Autodesk Inventor part; units mm, degrees
ref_plane "YZ Plane" through (0, 0, 0) normal (1, 0, 0) x (0, 1, 0)
ref_plane "XZ Plane" through (0, 0, 0) normal (0, 1, 0) x (-1, 0, 0)
ref_plane "XY Plane" through (0, 0, 0) normal (0, 0, 1) x (1, 0, 0)
sketch "Sketch1" plane through (0, 0, 0) normal (0, 0, 1) x (1, 0, 0)
  line L0 (50, -70) -> (50, 25)
  line L1 (-50, 25) -> (-50, -70)
  line L2 (0, 0) -> (-38.1854, 57.2781) construction
  arc A0 (50, 25) -> (-50, 25) centre (0, 25) ccw
  line L3 (-45, -90) -> (45, -90)
  line L4 (0, 0) -> (38.1854, 57.2781) construction
  line L5 (50, -70) -> (50, -85)
  line L6 (-50, -70) -> (-50, -85)
  arc A1 (45, -90) -> (50, -85) centre (45, -85) ccw
  arc A2 (-50, -85) -> (-45, -90) centre (-45, -85) ccw
  dimension "d19" = 5
extrude "Extrusion1" add sketch "Sketch1" along normal blind 47.5
shell "Shell1" thickness 2.5 removed faces 1 at (-16.6667, -6.6667, 0)
sketch "Sketch2" plane through (0, 25, 45) normal (0, 0, -1) x (-1, 0, 0)
  arc A0 (50, 0) -> (-50, 0) centre (0, 0) ccw
  line L0 (25, 0) -> (50, 0) construction
  line L1 (25, 0) -> (50, 0) construction
  line L2 (-25, 0) -> (-50, 0)
  line L3 (-47.5, -110) -> (-47.5, 0)
  line L4 (25, 0) -> (50, 0) construction
  line L5 (25, 0) -> (50, 0) construction
  line L6 (47.5, 0) -> (47.5, -112.5)
  line L7 (47.5, -112.5) -> (-47.5, -112.5)
  line L8 (-47.5, -112.5) -> (-47.5, 0)
  line L9 (20.5, -24.5) -> (29.5, -24.5)
  line L10 (29.5, -24.5) -> (29.5, -15.5)
  line L11 (29.5, -15.5) -> (20.5, -15.5)
  line L12 (20.5, -15.5) -> (20.5, -24.5)
  circle A1 centre (25, -20) radius 0.7
  line L13 (20.5, -24.5) -> (29.5, -15.5) construction
  line L14 (29.5, -24.5) -> (20.5, -15.5) construction
  circle A2 centre (36.5, -1.2321) radius 0.9
  line L15 (34.5, 0.7679) -> (38.5, 0.7679)
  line L16 (38.5, -3.2321) -> (34.5, -3.2321)
  line L17 (34.5, 0.7679) -> (38.5, -3.2321) construction
  line L18 (38.5, 0.7679) -> (34.5, -3.2321) construction
  line L19 (34.5, -3.2321) -> (34.5, 0.7679)
  line L20 (29.5, -15.5) -> (29.5, -24.5)
  circle A3 centre (25, -20) radius 0.7
  line L21 (20.5, -15.5) -> (29.5, -15.5)
  line L22 (29.5, -24.5) -> (20.5, -24.5)
  line L23 (20.5, -24.5) -> (20.5, -15.5)
  line L24 (20.5, -15.5) -> (29.5, -24.5) construction
  line L25 (29.5, -15.5) -> (20.5, -24.5) construction
  line L26 (11.5, -30.9599) -> (38.5, -30.9599)
  line L27 (38.5, 9.0401) -> (11.5, 9.0401)
  line L28 (11.5, 9.0401) -> (11.5, -30.9599)
  line L29 (38.5, -30.9599) -> (38.5, 9.0401)
  line L30 (38.5, 0.7679) -> (38.5, -3.2321)
  line L31 (25, -20) -> (25, 0)
  line L32 (-25, 0) -> (-25, -20)
  line L33 (-25, 0) -> (-5, 0) construction
  line L34 (-41, -30) -> (-9, -30)
  line L35 (-9, -30) -> (-9, -10)
  line L36 (-9, -10) -> (-41, -10)
  line L37 (-41, -10) -> (-41, -30)
  line L38 (-41, -30) -> (-9, -10) construction
  line L39 (-9, -30) -> (-41, -10) construction
  line L40 (0, 0) -> (0, 20)
  circle A4 centre (0, 20) radius 9.5
  line L41 (33.5, -108) -> (-35.5, -108)
  line L42 (-35.5, -108) -> (-35.5, -32)
  line L43 (-35.5, -32) -> (33.5, -32)
  line L44 (33.5, -32) -> (33.5, -108)
  line L45 (33.5, -108) -> (-35.5, -32) construction
  line L46 (-35.5, -108) -> (33.5, -32) construction
  line L47 (-15, -112) -> (15, -112)
  line L48 (15, -112) -> (15, -108)
  line L49 (15, -108) -> (-15, -108)
  line L50 (-15, -108) -> (-15, -112)
  line L51 (-15, -112) -> (15, -108) construction
  line L52 (15, -112) -> (-15, -108) construction
  point P0 (0, -25)
  point P1 (-47.5, -95)
  point P2 (25, -20)
  point P3 (-1, -70)
  point P4 (0, -110)
  dimension "d26" = 20
  dimension "d27" = 90
  dimension "d28" = 32
  dimension "d29" = 20
  dimension "d30" = 20
  dimension "d31" = 19
  dimension "d32" = 69
  dimension "d33" = 76
extrude "Extrusion2" cut sketch "Sketch2" against normal blind 50 contours A1 | L12 L11 L10 L9 | A2 | L15 L29 L16 L19 | L37 L36 L35 L34 | A4 | L48 L47 L50 L41
sketch "Sketch3" plane through (0, 25, 45) normal (0, 0, -1) x (-1, 0, 0)
  line L0 (29.5, -24.5) -> (29.5, -15.5)
  circle A0 centre (25, -20) radius 0.7
  line L1 (20.5, -24.5) -> (29.5, -24.5)
  line L2 (29.5, -15.5) -> (20.5, -15.5)
  line L3 (20.5, -15.5) -> (20.5, -24.5)
  line L4 (20.5, -24.5) -> (29.5, -15.5) construction
  line L5 (29.5, -24.5) -> (20.5, -15.5) construction
  circle A1 centre (36.5, -1.2321) radius 0.9
  line L6 (34.5, 0.7679) -> (38.5, -3.2321) construction
  circle A2 centre (25, -20) radius 0.7
  line L7 (20.5, -15.5) -> (29.5, -15.5)
  line L8 (29.5, -15.5) -> (29.5, -24.5)
  line L9 (29.5, -24.5) -> (20.5, -24.5)
  line L10 (20.5, -24.5) -> (20.5, -15.5)
  line L11 (20.5, -15.5) -> (29.5, -24.5) construction
  line L12 (29.5, -15.5) -> (20.5, -24.5) construction
  line L13 (38.5, -3.2321) -> (34.5, -3.2321)
  line L14 (34.5, -3.2321) -> (34.5, 0.7679)
  line L15 (38.5, 0.7679) -> (38.5, -3.2321)
  line L16 (38.5, 0.7679) -> (34.5, -3.2321) construction
  line L17 (34.5, 0.7679) -> (38.5, 0.7679)
  line L18 (11.5, -30.9599) -> (38.5, -30.9599)
  line L19 (11.5, 9.0401) -> (11.5, -30.9599)
  line L20 (38.5, -30.9599) -> (38.5, 9.0401)
  line L21 (38.5, 9.0401) -> (11.5, 9.0401)
  line L22 (25, -20) -> (25, 0)
  line L23 (-25, 0) -> (-25, -20)
  line L24 (-25, 0) -> (-5, 0) construction
  line L25 (-41, -30) -> (-9, -30)
  line L26 (-9, -30) -> (-9, -10)
  line L27 (-9, -10) -> (-41, -10)
  line L28 (-41, -10) -> (-41, -30)
  line L29 (-41, -30) -> (-9, -10) construction
  line L30 (-9, -30) -> (-41, -10) construction
  line L31 (0, 0) -> (0, 20)
  line L32 (9.5, -32.9599) -> (40.5, -32.9599)
  line L33 (40.5, -32.9599) -> (40.5, 11.0401)
  line L34 (40.5, 11.0401) -> (9.5, 11.0401)
  line L35 (9.5, 11.0401) -> (9.5, -32.9599)
  line L36 (-7, -8) -> (-7, -32)
  line L37 (-43, -32) -> (-43, -8)
  line L38 (-41, -30) -> (-41, -32)
  line L39 (11.25, 9.2901) -> (38.75, 9.2901)
  line L40 (38.75, 9.2901) -> (38.75, -31.2099)
  line L41 (38.75, -31.2099) -> (11.25, -31.2099)
  line L42 (11.25, -31.2099) -> (11.25, 9.2901)
  line L43 (-25, -9.75) -> (-8.75, -9.75)
  line L44 (-8.75, -9.75) -> (-8.75, -30.25)
  line L45 (-8.75, -30.25) -> (-41.25, -30.25)
  line L46 (-41.25, -30.25) -> (-41.25, -9.75)
  line L47 (-41.25, -9.75) -> (-41.25, -8)
  line L48 (-41.25, -30.25) -> (-41.25, -32)
  line L49 (-8.75, -30.25) -> (-8.75, -32)
  line L50 (-8.75, -9.75) -> (-8.75, -8)
  line L51 (-43, -8) -> (-41.25, -8)
  line L52 (-8.75, -8) -> (-7, -8)
  line L53 (-7, -32) -> (-8.75, -32)
  line L54 (-41, -32) -> (-43, -32)
  line L55 (6, -20.0179) -> (44, -20.0179)
  line L56 (44, -20.0179) -> (44, 2.2679)
  line L57 (44, 2.2679) -> (6, 2.2679)
  line L58 (6, 2.2679) -> (6, -20.0179)
  line L59 (6, -20.0179) -> (44, 2.2679) construction
  line L60 (44, -20.0179) -> (6, 2.2679) construction
  point P0 (0, -25)
  point P1 (25, -20)
  point P2 (25, -8.875)
  point P3 (40.5, -20.0179)
  point P4 (38.75, -20.0179)
  point P5 (11.25, -20.0179)
  point P6 (9.5, -20.0179)
  point P7 (9.5, 2.2679)
  point P8 (11.25, 2.2679)
  point P9 (38.75, 2.2679)
  point P10 (40.5, 2.2679)
  dimension "d36" = 20
  dimension "d37" = 90
  dimension "d39" = 20
  dimension "d40" = 20
  dimension "d41" = 2
  dimension "d42" = 0.25
  dimension "d44" = 0.25
extrude "Extrusion3" add sketch "Sketch3" along normal blind 10 contours L55 L33 L32 L35 L42 L41 L40 | L40 L39 L42 L57 L35 L34 L33 | L50 L52 L36 L53 L49 L44 | L48 L54 L37 L51 L47 L46
chamfer "Chamfer1" distance 1 angle 45 12 edges at (25, 15, 47.5) (41, 5, 47.5) (25, -5, 47.5) (9, 5, 47.5) (-25, 9.5, 47.5) (-20.5, 5, 47.5) (-29.5, 5, 47.5) (-25, 0.5, 47.5) (-36.5, 21.7679, 47.5) (-34.5, 23.7679, 47.5) (-36.5, 25.7679, 47.5) (-38.5, 23.7679, 47.5)
chamfer "Chamfer2" distance 1 angle 45 4 edges at (0, -83, 47.5) (0, -87, 47.5) (-15, -85, 47.5) (15, -85, 47.5)
sketch "Sketch4" plane through (0, 0, 47.5) normal (0, 0, 1) x (1, 0, 0)
  line L0 (15, -83) -> (-15, -83)
  line L1 (0, -83) -> (0, -45)
  line L2 (-35, -83.5) -> (35, -83.5)
  line L3 (35, -83.5) -> (35, -6.5)
  line L4 (35, -6.5) -> (-35, -6.5)
  line L5 (-35, -6.5) -> (-35, -83.5)
  line L6 (-35, -83.5) -> (35, -6.5) construction
  line L7 (35, -83.5) -> (-35, -6.5) construction
  point P0 (0, 0)
  dimension "d53" = 38
  dimension "d54" = 70
  dimension "d55" = 77
extrude "Extrusion4" cut sketch "Sketch4" against normal blind 1
chamfer "Chamfer3" distance 1.5 angle 45 6 edges at (0, 75, 47.5) (-50, -30, 47.5) (-48.5355, -88.5355, 47.5) (0, -90, 47.5) (48.5355, -88.5355, 47.5) (50, -30, 47.5)
sketch "Sketch5" plane through (-45, -90, 0) normal (0, -1, 0) x (1, 0, 0)
  line L0 (45, 0) -> (45, 5)
  circle A0 centre (45, 2.5) radius 1.45
  dimension "d61" = 5
  dimension "d62" = 2.9
extrude "Extrusion5" cut sketch "Sketch5" against normal through all
properties part number "enclouser"
Could you check a few things on this model? Use its own coordinates, in mm. A direction names the side the tool comes from. Give positions to 0.01 mm unless a question says otherwise; leave off trailing zeros. Write each loop counter-clockwise with the first axis right and the second up, starting at its lowest first coordinate (ties: lowest second). Pieces come first, ordered by that corner, then holes. Notation, with made-up numbers: (25, -26) -> (48, -26) arc R10 ccw to (48, -12) -> close; hole circle Ø10 at (52, -34). An arc over 180 degrees is marked (long way). Answer as CSV lines item,"result". Start each with the question number.
(1) Which directions (+Z, -Z, +X, -X, +Y, -Y) give clear straight access to the entire face, cutting with the end or side of a thin tool? Please do faces 4 (the face through (-47.9, -87.9, 46.9)), 5 (the face through (0, -44, 46.5)), 6 (the face through (-9.5, 32, 40)).
(2) If we section it at B-B, the plane z = 38.5: Give the number of separate pieces and of enclosed holes in the cut face, and give its area (3 significant figures).
(3) If we section it at C-C, the plane y = -35: Write out the boundary of the cut face in (x, z).
(4) Please list where these lines run through material, in increasing order: line 1 (X direction, y = 11, z = 42.5); line 2 (Y direction, x = 0, z = 46); line 3 (X direction, y = -29, z = 27).
(5) If we mould it in two halves opening along X, with no side actions, what happens to faces 1 (the face through (-1.07, 73.75, 47.24)), 2 (the face through (-50, -29, 23)), 3 (the face through (-11.25, -1, 40))? For each: +X half, -X half, draft (parallel to the pull), parting line (faces both ways), or undercut.
(6) If we section it at A-A, the plane z = 18: Write out the boundary of the cut face in (x, y), and give its area (3 significant figures).
(7) I'm going to push flat-ended pins straight in: pin 1 Ø6 at (x, z) = (-17, 7.5) entering from +Y; pin 2 Ø1.5 at (x, y) = (28.5, -11.5) entering from -Z; pin 3 Ø2 at (x, z) = (3.5, 38.5) entering from +Y. Where does each tip first touch, or does it pass through?
Answer list:
1,face 4,"+Z, -X, -Y"
1,face 5,"+Z"
1,face 6,"-Z"
2,separate pieces,"5"
2,enclosed holes,"1"
2,area,"1,440 mm^2"
3,outline,"(-50, 0) -> (-47.5, 0) -> (-47.5, 45) -> (47.5, 45) -> (47.5, 0) -> (50, 0) -> (50, 46) -> (48.5, 47.5) -> (35, 47.5) -> (35, 46.5) -> (-35, 46.5) -> (-35, 47.5) -> (-48.5, 47.5) -> (-50, 46) -> close"
4,line 1,"-50 to -47.5, 7 to 8.75, 41.25 to 43, 47.5 to 50"
4,line 2,"-90 to -87, -83 to 35.5, 54.5 to 75"
4,line 3,"-50 to -47.5, 47.5 to 50"
5,face 1,"parting line"
5,face 2,"-X half"
5,face 3,"undercut"
6,outline,"(-50, -85) arc R5 ccw to (-45, -90) -> (45, -90) arc R5 ccw to (50, -85) -> (50, 25) arc R50 ccw to (-50, 25) -> close; hole (-47.5, -85) arc R2.5 ccw to (-45, -87.5) -> (45, -87.5) arc R2.5 ccw to (47.5, -85) -> (47.5, 25) arc R47.5 ccw to (-47.5, 25) -> close"
6,area,"1,190 mm^2"
7,pin 1,"y = 73"
7,pin 2,"z = 45"
7,pin 3,"y = 74.94"
